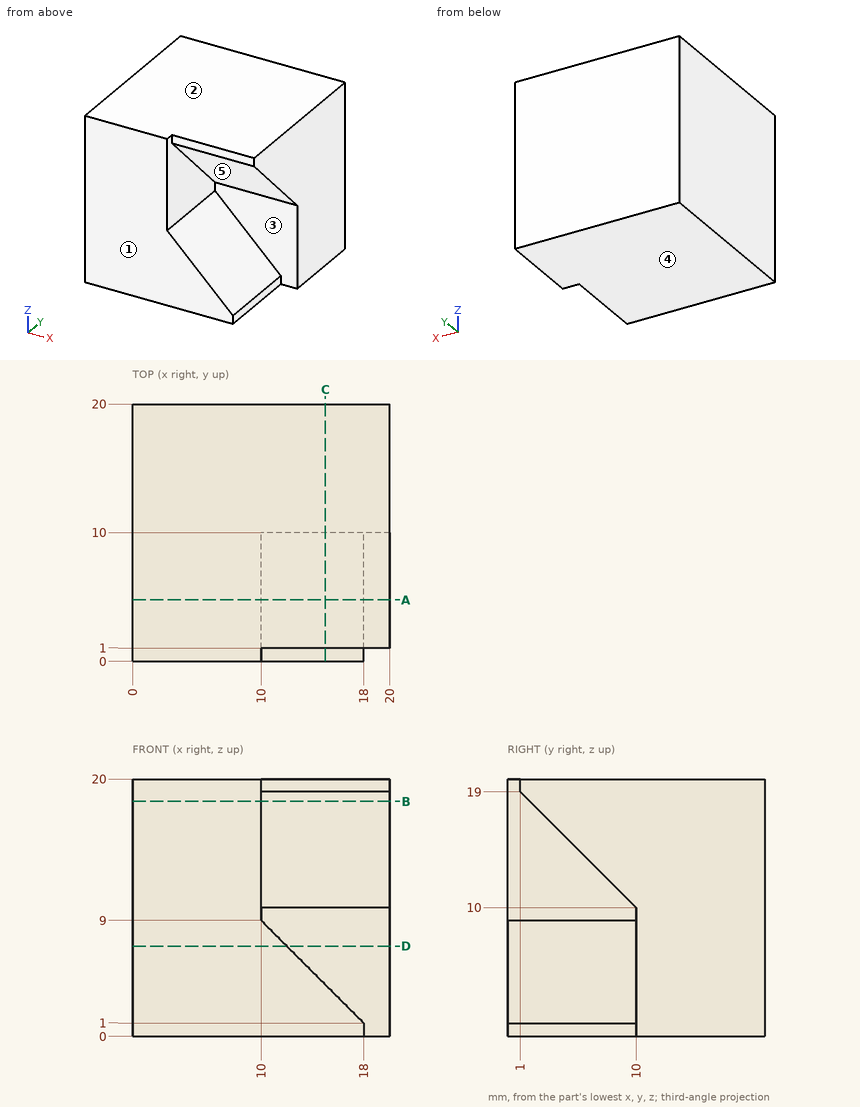
The figure shows three views and two pictorial views of one solid part (mm, origin at its lowest corner). Answer the questions. A direction names the side the tool comes from. Round coordinates to 2 decimals unless told otherwise and drop trailing zeros. Loops run counter-clockwise (first coordinate to the right, second up) from the corner with the lowest first, then second, coordinate; pieces in that order, holes last. Notation, with made-up numbers: M 20,-17.5 L 59,-17.5 A15 cw 59,-7.5 Z; hole C 68,30 d4. An arc over 180 degrees is marked long. Return JSON: item names as keys, results as strings.
Q1. Find section B-B, the plane z = 18.25. Determine the outline of the cut face in (x, y).
Results list:
{"outline": "M 0,0 L 10,0 L 10,1.75 L 20,1.75 L 20,20 L 0,20 Z"}
Q2. The mould has two halves that part along Z. Classify the marked faces 1, 2 and 3: released by +Z, released by -Z, zero draft, split by the parting line, or undercut.
Results list:
{"face 1": "zero draft", "face 2": "released by +Z", "face 3": "undercut"}
Q3. Which of the six approach directions +Z, -Z, +X, -X, +Y, -Y give full straight-line access (tool end or side, diameter ignored) to the marked faces 4 and 5?
Results list:
{"face 4": "-Z, +X, -X, +Y, -Y", "face 5": "+X, -Y"}
Q4. Each of these flat-tipped pins is pushed along its axis until it touches: pin 1 Ø4 at (y, z) = (2, 5) entering from +X; pin 2 Ø0.5 at (y, z) = (7, 0.5) entering from +X. Where does it stop, or does it pass through?
Results list:
{"pin 1": "stops at x = 16", "pin 2": "stops at x = 18"}
Q5. Find the intervals of material crossed by line 1 along Z through (x, y) = (14, 7.5); line 2 along X through (y, z) = (2.5, 14.5); line 3 along Z through (x, y) = (16.5, 7), in increasing order. Write a range as from..to.
Results list:
{"line 1": "z = 0..5, 12.5..20", "line 2": "x = 0..10", "line 3": "z = 0..2.5, 13..20"}
Q6. Find section A-A, the plane y = 4.75. Determine the outline of the cut face in (x, z), plus the area to 4 significant figures.
Results list:
{"outline": "M 0,0 L 18,0 L 18,1 L 10,9 L 10,15.25 L 20,15.25 L 20,20 L 0,20 Z", "area": "287.5 mm2"}
Q7. Find section C-C, the plane x = 15. Determine the outline of the cut face in (y, z), plus the area to 4 significant figures.
Results list:
{"outline": "M 0,0 L 20,0 L 20,20 L 1,20 L 1,19 L 10,10 L 10,4 L 0,4 Z", "area": "289.5 mm2"}
Q8. Find section D-D, the plane z = 7. Determine the outline of the cut face in (x, y).
Results list:
{"outline": "M 0,0 L 12,0 L 12,10 L 20,10 L 20,20 L 0,20 Z"}
